```python
from build123d import *

# Parameters (mm, degrees)
SALIENTE_EXTRUIR1_DEPTH = 10
CROQUIS2_R              = 8.05
CROQUIS2_R_2            = 4
CORTAR_EXTRUIR1_DEPTH   = 10
CROQUIS3_R              = 10
SALIENTE_EXTRUIR2_DEPTH = 3
SALIENTE_EXTRUIR3_START = 3
CROQUIS4_R              = 10
SALIENTE_EXTRUIR3_DEPTH = 3
CROQUIS5_R              = 6.25
CORTAR_EXTRUIR2_DEPTH   = 59.14636704


with BuildPart() as part:
    # Croquis1 → Saliente-Extruir1 (new body)
    with BuildSketch(Plane(origin=(0, 0, 0), x_dir=(1, 0, 0), z_dir=(0, 1, 0))):
        with BuildLine():
            ThreePointArc((-8.111620656, 5.848214286), (-7.783099854, -6.278802168), (4, -9.16515139))
            ThreePointArc((4, -9.16515139), (14, -7.078029865), (24, -9.16515139))
            ThreePointArc((24, -9.16515139), (37.413063718, -3.375534245), (30.735830721, 9.618483782))
            ThreePointArc((30.735830721, 9.618483782), (18.80756088, 17.149005774), (12.854744679, 29.937921371))
            ThreePointArc((12.854744679, 29.937921371), (-5.873008246, 39.597748667), (-9.169658133, 18.784937888))
            ThreePointArc((-9.169658133, 18.784937888), (-6.25651887, 12.511562773), (-8.111620656, 5.848214286))
        make_face()
    extrude(amount=SALIENTE_EXTRUIR1_DEPTH)

    # Croquis2 → Cortar-Extruir1 (cut)
    with BuildSketch(Plane(origin=(0, 10, 0), x_dir=(1, 0, 0), z_dir=(0, 1, 0))):
        with Locations(Location((0, 28, 0), (0, 0, 270))):
            Circle(CROQUIS2_R)
        with Locations(Location((28, 0, 0), (0, 0, 270))):
            Circle(CROQUIS2_R_2)
    extrude(amount=-CORTAR_EXTRUIR1_DEPTH, mode=Mode.SUBTRACT)

    # Croquis3 → Saliente-Extruir2 (add)
    with BuildSketch(Plane(origin=(0, 10, 0), x_dir=(1, 0, 0), z_dir=(0, 1, 0))):
        with Locations(Location((0, 0, 0), (0, 0, 144.209624239))):
            Circle(CROQUIS3_R)
    extrude(amount=SALIENTE_EXTRUIR2_DEPTH)

    # Croquis4 → Saliente-Extruir3 (add)
    with BuildSketch(Plane.XZ.offset(SALIENTE_EXTRUIR3_START)):
        with Locations(Location((0, 0, 0), (0, 0, 270))):
            Circle(CROQUIS4_R)
    extrude(amount=-SALIENTE_EXTRUIR3_DEPTH)

    # Croquis5 → Cortar-Extruir2 (cut, through all)
    with BuildSketch(Plane(origin=(0, 13, 0), x_dir=(1, 0, 0), z_dir=(0, 1, 0))):
        with Locations(Location((0, 0, 0), (0, 0, 270))):
            Circle(CROQUIS5_R)
    extrude(amount=-CORTAR_EXTRUIR2_DEPTH, mode=Mode.SUBTRACT)


solid = part.part
```
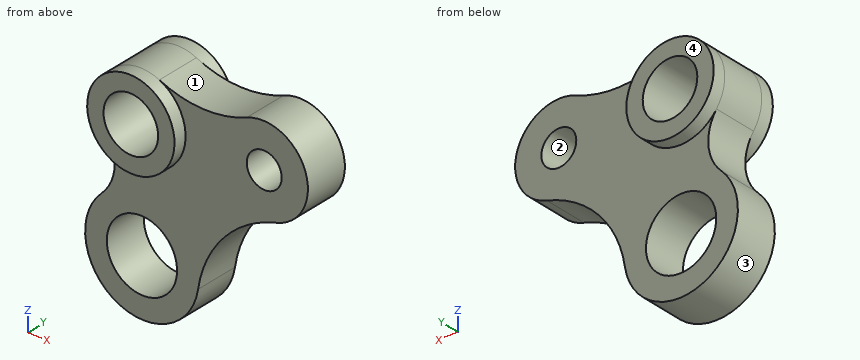
Check sheet for the modelled part. Datum: model origin and axes. Units: mm. Face numbers are marked on the shaded views. Give positions to 0.01 mm unless a question says otherwise; leave off trailing zeros. Order: outer loops, then holes, each group sorted by start corner. A loop starts at its lowest first (then second) coordinate and runs counter-clockwise, first axis right, second up. Notation, with made-up numbers: M 84,19.25 L 120,19.25 A3 cw 120,24.25 Z; hole C 20,6 d4. An arc over 180 degrees is marked long. Answer in a Markdown table with one row per item. Add a question column.
Q1. Sectioned sample at B-B, the plane x = 28. Record the boundary of the cut face in (y, z).
Q2. Sectioned sample at A-A, the plane z = 0. Record the boundary of the cut face in (x, y), and give its area (3 significant figures).
Q3. Sectioned sample at C-C, the plane x = 0. Record the boundary of the cut face in (y, z).
Q4. Sectioned sample at D-D, the plane y = 1. Record the boundary of the cut face in (x, z), and give its area (3 significant figures).
Q5. Gauge pin test, flat ends, axial feed: pin 1 Ø18.5 at (x, z) = (0, -28) entering from -Y; pin 2 Ø2 at (x, z) = (14.5, 0) entering from +Y; pin 3 Ø4 at (x, y) = (16.5, 0.5) entering from -Z. Record the tip position at first contact, or that the pin passes through.
Q6. Thickness scan on L1, parallel to X at y = 2.5, z = 0; L2, parallel to Y at x = 20, z = -14; L3, parallel to X at y = 8.5, z = -32. Record the ranges inside material, lowest first.
Q7. Release check for a two-part mould opening along X. For the marked faces 1, 2, 3 and 4 record: released by +X, released by -X, zero draft, split by the parting line, or undercut.
Verdict:
| question | item | result |
|---|---|---|
| 1 | outline | M 0,-10.57 L 10,-10.57 L 10,-4 L 0,-4 Z; M 0,4 L 10,4 L 10,10 L 0,10 Z |
| 2 | outline | M -10,-3 L -6.25,-3 L -6.25,13 L -10,13 Z; M 6.25,-3 L 10,-3 L 10,0 L 24,0 L 24,10 L 10,10 L 10,13 L 6.25,13 Z; M 32,0 L 38,0 L 38,10 L 32,10 Z |
| 2 | area | 320 mm² |
| 3 | outline | M -3,-10 L 0,-10 L 0,-19.95 L 10,-19.95 L 10,-10 L 13,-10 L 13,-6.25 L -3,-6.25 Z; M -3,6.25 L 13,6.25 L 13,10 L -3,10 Z; M 0,-41 L 10,-41 L 10,-36.05 L 0,-36.05 Z |
| 4 | outline | M -9.17,-18.78 A13 ccw long 12.85,-29.94 A25 cw 30.74,-9.62 A10 ccw long 24,9.17 A25 cw 4,9.17 A10 ccw -8.11,-5.85 A10 cw Z; hole C 0,-28 d16.1; hole C 0,0 d12.5; hole C 28,0 d8 |
| 4 | area | 1,230 mm² |
| 5 | pin 1 | y = 0 |
| 5 | pin 2 | y = 10 |
| 5 | pin 3 | z = -24.05 |
| 6 | L1 | -10 to -6.25, 6.25 to 24, 32 to 38 |
| 6 | L2 | 0 to 10 |
| 6 | L3 | -12.37 to -6.99, 6.99 to 12.37 |
| 7 | face 1 | undercut |
| 7 | face 2 | undercut |
| 7 | face 3 | split by the parting line |
| 7 | face 4 | zero draft |
